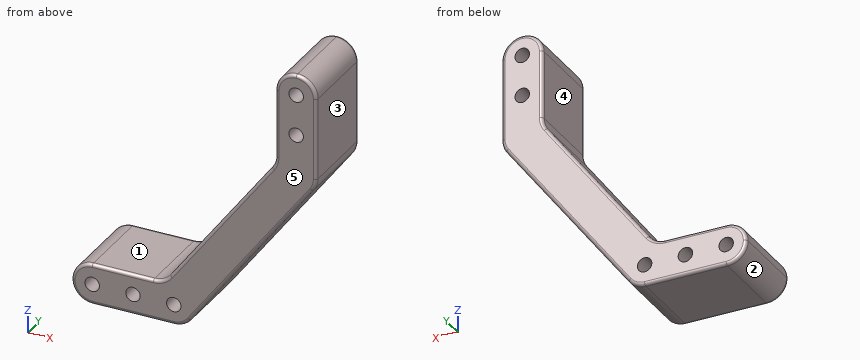
```python
from build123d import *

# Parameters (mm, degrees)
SKETCH1_R           = 2.25
BOSS_EXTRUDE1_DEPTH = 25.4
FILLET1_R           = 6.35
FILLET2_R           = 1


with BuildPart() as part:
    # Sketch1 → Boss-Extrude1 (new body)
    with BuildSketch(Plane(origin=(0, 0, 0), x_dir=(1, 0, 0), z_dir=(0, 1, 0))):
        Polygon((-6.35, 6.35), (-6.35, -6.35), (22.225, -6.35), (57.15, -52.916666667), (57.15, -82.55), (69.85, -82.55), (69.85, -48.683333333), (28.575, 6.35), align=None)
        with Locations(Location((0, 0, 0), (0, 0, 270))):
            Circle(SKETCH1_R, mode=Mode.SUBTRACT)
        with Locations(Location((63.5, -76.2, 0), (0, 0, 270))):
            Circle(SKETCH1_R, mode=Mode.SUBTRACT)
        with Locations(Location((63.5, -63.5, 0), (0, 0, 270))):
            Circle(SKETCH1_R, mode=Mode.SUBTRACT)
        with Locations(Location((12.7, 0, 0), (0, 0, 270))):
            Circle(SKETCH1_R, mode=Mode.SUBTRACT)
        with Locations(Location((25.4, 0, 0), (0, 0, 270))):
            Circle(SKETCH1_R, mode=Mode.SUBTRACT)
    extrude(amount=BOSS_EXTRUDE1_DEPTH)

    # Fillet1
    fillet1_edges = [part.edges().sort_by_distance(p)[0] for p in [
        (28.575, 12.7, -6.35),
        (22.225, 12.7, 6.35),
        (69.85, 12.7, 48.683333333),
        (57.15, 12.7, 52.916666667),
        (69.85, 12.7, 82.55),
        (57.15, 12.7, 82.55),
        (-6.35, 12.7, -6.35),
        (-6.35, 12.7, 6.35),
    ]]
    fillet(fillet1_edges, radius=FILLET1_R - 0.0001)  # a hair under: the kernel refuses the full size

    # Fillet2
    fillet2_edges = [part.edges().sort_by_distance(p)[0] for p in [
        (12.699975, 0, -6.35),
        (12.699975, 25.4, -6.35),
        (49.529995, 0, 21.589993333),
        (69.85, 0, 63.500033333),
        (57.15, 0, 65.6167),
        (40.004995, 0, 30.05666),
        (9.524975, 0, 6.35),
        (-4.49015735, 0, 4.49015735),
        (-4.49015735, 0, -4.49015735),
        (59.00984265, 0, 80.69015735),
        (67.99015735, 0, 80.69015735),
        (69.524144074, 0, 48.791951975),
        (28.23981161, 0, -5.67962322),
        (49.529995, 25.4, 21.589993333),
        (9.524975, 25.4, 6.35),
        (40.004995, 25.4, 30.05666),
        (57.15, 25.4, 65.6167),
        (69.85, 25.4, 63.500033333),
        (-4.49015735, 25.4, 4.49015735),
        (-4.49015735, 25.4, -4.49015735),
        (59.00984265, 25.4, 80.69015735),
        (67.99015735, 25.4, 80.69015735),
        (69.524144074, 25.4, 48.791951975),
        (28.23981161, 25.4, -5.67962322),
        (21.88981161, 0, 7.02037678),
        (21.88981161, 25.4, 7.02037678),
        (56.824144074, 0, 53.025285309),
        (56.824144074, 25.4, 53.025285309),
    ]]
    fillet(fillet2_edges, radius=FILLET2_R)


solid = part.part
```
Part model, mm, in its own coordinate system. Face numbers are marked on the shaded views. A direction names the side the tool comes from. Give positions to 0.01 mm unless a question says otherwise; leave off trailing zeros. Loops run counter-clockwise (first coordinate to the right, second up) from the corner with the lowest first, then second, coordinate; pieces in that order, holes last. Notation, with made-up numbers: M 86,-23.75 L 96,-23.75 A29 ccw 96,-3.75 Z; hole C -4.5,33 d5. An arc over 180 degrees is marked long. Return JSON: item names as keys, results as strings.
1) Saw through at B-B, the plane z = 63.5. List the corners of the cut face in (x, y).
Calculated:
{"outline": "M 57.15,1 A1 ccw 58.15,0 L 61.25,0 L 61.25,25.4 L 58.15,25.4 A1 ccw 57.15,24.4 Z; M 65.75,0 L 68.85,0 A1 ccw 69.85,1 L 69.85,24.4 A1 ccw 68.85,25.4 L 65.75,25.4 Z"}
2) 3-axis set-ups, long thin cutter, end or side, ignore diameter. For the marked faces 4 and 5: which of +Z, -Z, +X, -X, +Y, -Y reach the whole face in a straight line?
Calculated:
{"face 4": "+Z, -X, +Y, -Y", "face 5": "+Z, -Z, +X, -X, -Y"}
3) Pull direction Z, two halves, no side cores. Call the marked faces 1, 2 and 3: released by +Z, released by -Z, zero draft, split by the parting line, or undercut.
Calculated:
{"face 1": "released by +Z", "face 2": "released by -Z", "face 3": "zero draft"}
4) Flat gauge pins, fed straight in: pin 1 Ø12 at (y, z) = (8, 43.5) entering from +X; pin 2 Ø3 at (x, y) = (41, 7.5) entering from +Z; pin 3 Ø1.5 at (x, y) = (49, 9) entering from -Z. Where does each tip first touch, or does it go through?
Calculated:
{"pin 1": "stops at x = 69.72", "pin 2": "stops at z = 33.38", "pin 3": "stops at z = 19.88"}
5) Saw through at C-C, the plane y = 12.25. Count the separate pieces of the cut face and the enclosed holes in it, then the cut area to 3 significant figures.
Calculated:
{"separate pieces": "1", "enclosed holes": "5", "area": "1,500 mm2"}
6) Drill centre lines: line 1 (X direction, y = 20.5, z = 0); line 2 (X direction, y = 18.25, z = 76.2); line 3 (X direction, y = 7, z = 70.5). Where is each one in solid material? Low to high.
Calculated:
{"line 1": "x = -6.35 to -2.25, 2.25 to 10.45, 14.95 to 23.15, 27.65 to 33.34", "line 2": "x = 57.15 to 61.25, 65.75 to 69.85", "line 3": "x = 57.15 to 69.85"}
7) Saw through at A-A, the plane x = 12.7. List the corners of the cut face in (y, z).
Calculated:
{"outline": "M 0,-5.35 A1 ccw 1,-6.35 L 24.4,-6.35 A1 ccw 25.4,-5.35 L 25.4,-2.25 L 0,-2.25 Z; M 0,2.25 L 25.4,2.25 L 25.4,5.35 A1 ccw 24.4,6.35 L 1,6.35 A1 ccw 0,5.35 Z"}
